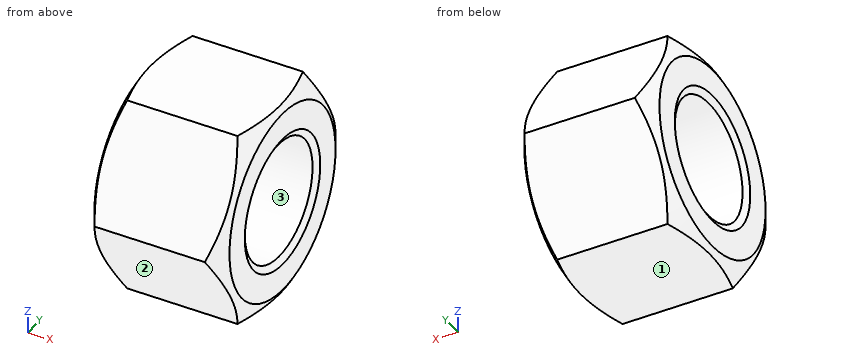
Autodesk Inventor part; units mm, degrees
ref_plane "Work Plane1" through (-24.1737, 0, 0) normal (0, -0.866, -0.5) x (1, 0, 0)
ref_plane "YZ Plane" through (0, 0, 0) normal (1, 0, 0) x (0, 1, 0)
ref_plane "XZ Plane" through (0, 0, 0) normal (0, 1, 0) x (-1, 0, 0)
sketch "Sketch1" plane through (0, 0, 0) normal (1, 0, 0) x (0, 1, 0)
  line L0 (-13.8564, 0) -> (-6.9282, 12)
  line L1 (-6.9282, 12) -> (6.9282, 12)
  line L2 (6.9282, 12) -> (13.8564, 0)
  line L3 (13.8564, 0) -> (6.9282, -12)
  line L4 (6.9282, -12) -> (-6.9282, -12)
  line L5 (-6.9282, -12) -> (-13.8564, 0)
  point P0 (0, 0)
  point P1 (0, 0)
  dimension "d0" = 27.7128
extrude "Body" add sketch "Sketch1" along normal blind 16.4
sketch "Sketch2" plane through (0, 0, 0) normal (0, 0, 1) x (1, 0, 0)
  line L0 (0, 6.9282) -> (0, 13.8564)
  line L1 (0, 13.8564) -> (16.4, 13.8564)
  line L2 (16.4, 6.9282) -> (16.4, 13.8564)
  line L3 (-3.28, 0) -> (19.68, 0)
  line L4 (1.5077, 13.8564) -> (0, 11.245)
  line L5 (14.8923, 13.8564) -> (16.4, 11.245)
  dimension "d3" = 30
  dimension "d4" = 30
  dimension "d5" = 22.49
  dimension "d6" = 22.49
revolve "Chamfer1" cut sketch "Sketch2" angle 360 about axis through (-10, 0, 0) along (1, 0, 0)
sketch "Sketch3" plane through (16.4, 0, 0) normal (1, 0, 0) x (0, 0, -1)
  arc A0 (-0.625, -1.0825) -> (0.625, -1.0825) centre (0, 0) ccw
hole "Thread" at (16.4, 0, 0) direction (-1, 0, 0) diameter 14.376 end through all
chamfer "Chamfer2" distance 0.8119 angle 30 1 edges at (16.4, 0, 7.188) measured on face at (16.4, 9.7663, -1.1858)
chamfer "Chamfer3" distance 0.8119 angle 30 1 edges at (0, 0, 7.188) measured on face at (0, 9.7663, -1.1858)
ref_plane "Work Plane1" through (-24.1737, 0, 0) normal (0, -0.866, -0.5) x (1, 0, 0)
equation "\"d0\" = 1.1547 * SW"
equation "\"d1\" = KOH"
equation "\"d8\" = -0.5 * GD1 + 0.5 * NND"
equation "\"d40\" = -0.5 * GD1 + 0.5 * NND"
equation "\"d10\" = -0.5 * GD1 + 0.5 * NND"
equation "\"d41\" = -0.5 * GD1 + 0.5 * NND"
equation "\"d3\" = ANG1"
equation "\"d4\" = ANG2"
equation "\"d5\" = SW0"
equation "\"d6\" = SW01"
equation "\"ANG1\" = 30deg"
equation "\"ANG2\" = 30deg"
equation "\"NND\" = 16"
equation "\"KOH\" = 16.4"
equation "\"SW\" = 24"
equation "\"SW0\" = 22.49"
equation "\"SW01\" = SW0"
equation "\"GUL\" = 0.541266 * PTC"
equation "\"THREADDIA\" = 16"
equation "\"TOA\" = 30deg"
equation "\"PTC\" = 1.5"
equation "\"E0\" = 26.75"
equation "\"GAL\" = 0.541266 * PTC"
equation "\"KOH1\" = 12.56"
properties part number "ISO 8674 - M16 x 1,5" material "Steel"
For this review, take the finished solid that the model builds, in its own axes (mm). Face numbers are marked on the shaded views. Give positions to 0.01 mm unless a question says otherwise; leave off trailing zeros. Order: outer loops, then holes, each group sorted by start corner. A loop starts at its lowest first (then second) coordinate and runs counter-clockwise, first axis right, second up.
1) The part is to be moulded in two halves that separate along Y. For the marked faces 1, 2 and 3, say which applies: released by +Y, released by -Y, zero draft, split by the parting line, or undercut.
2) Wall thickness on line 1 (Z direction, x = 12, y = 0); line 2 (Y direction, x = 12.75, z = 5); line 3 (Z direction, x = 6.75, y = 3): over which ranges is each line inside the solid? List them lowest first.
3) Take a section at B-B (x = 10). Give the boundary of the cut face in (y, z), then the cut area to 3 significant figures.
4) Take a section at A-A (y = 0). Give the boundary of the cut face in (x, z) (3 decimals), then the cut area to 3 significant figures.
Derived:
1. face 1: zero draft
1. face 2: released by -Y
1. face 3: undercut
2. line 1: z = -12 to -7.19, 7.19 to 12
2. line 2: y = -10.97 to -5.16, 5.16 to 10.97
2. line 3: z = -12 to -6.53, 6.53 to 12
3. outline: (-13.86, 0) - (-6.93, -12) - (6.93, -12) - (13.86, 0) - (6.93, 12) - (-6.93, 12) - close; hole circle Ø14.38 at (0, 0)
3. area: 337 mm2
4. outline: (0, -11.245) - (0.436, -12) - (15.964, -12) - (16.4, -11.245) - (16.4, -8) - (15.931, -7.188) - (0.469, -7.188) - (0, -8) - close; (0, 8) - (0.469, 7.188) - (15.931, 7.188) - (16.4, 8) - (16.4, 11.245) - (15.964, 12) - (0.436, 12) - (0, 11.245) - close
4. area: 156 mm2
